from build123d import *

# Parameters (mm, degrees)
CROQUIS1_R                   = 275
SALIENTE_EXTRUIR1_DEPTH      = 70
CROQUIS2_R                   = 200
CORTAR_EXTRUIR1_DEPTH        = 40
CROQUIS5_R                   = 10
CORTAR_EXTRUIR2_DEPTH        = 10
REDONDEO1_R                  = 2
CORTAR_EXTRUIR_L_MINA2_DEPTH = 396.15819617
MATRIZC1_COUNT               = 24
CORTAR_EXTRUIR3_DEPTH        = 150
SALIENTE_EXTRUIR2_DEPTH      = 50
SALIENTE_EXTRUIR2_DEPTH_BACK = 50
CROQUIS12_R                  = 19.934957438
CROQUIS14_R                  = 285.546784005
CROQUIS14_R_2                = 202
SALIENTE_EXTRUIR3_DEPTH      = 100
REDONDEO2_R                  = 30
REDONDEO3_R                  = 30
SCALE1_SCALE                 = 0.5
SCALE2_SCALE                 = 0.1
SCALE3_SCALE                 = 0.2
SCALE4_SCALE                 = 0.3
SCALE5_SCALE                 = 20
SCALE6_SCALE                 = 1.5
SKETCH1_R                    = 1
CUT_EXTRUDE1_DEPTH           = 5


with BuildPart() as part:
    # Croquis1 → Saliente-Extruir1 (new body)
    with BuildSketch(Plane.XY):
        Circle(CROQUIS1_R)
    extrude(amount=SALIENTE_EXTRUIR1_DEPTH)

    # Croquis2 → Cortar-Extruir1 (cut)
    with BuildSketch(Plane.XY.offset(70)):
        Circle(CROQUIS2_R)
    extrude(amount=-CORTAR_EXTRUIR1_DEPTH, mode=Mode.SUBTRACT)

    # Croquis5 → Cortar-Extruir2 (cut)
    with BuildSketch(Plane.XY.offset(30)):
        Circle(CROQUIS5_R)
    extrude(amount=-CORTAR_EXTRUIR2_DEPTH, mode=Mode.SUBTRACT)

    # Redondeo1
    redondeo1_edges = [part.edges().sort_by_distance(p)[0] for p in [
        (-200, 0, 70),
    ]]
    fillet(redondeo1_edges, radius=REDONDEO1_R)

    # Croquis6 → Cortar-Extruir-Lámina2 (cut, through all)
    with BuildSketch(Plane.XY.offset(70)):
        Polygon((-99.341458201, 256.429863086), (-89.226691548, 230.320640663), (-89.319938771, 230.284516496), (-99.434705424, 256.39373892), align=None)
    cortar_extruir_l_mina2 = extrude(amount=-CORTAR_EXTRUIR_L_MINA2_DEPTH, mode=Mode.SUBTRACT)

    # MatrizC1: Cortar-Extruir-Lámina2 ×24 about axis
    matrizc1_axis = Axis((0, 0, 0), (0, 0, 1))
    for i in range(1, MATRIZC1_COUNT):
        add(cortar_extruir_l_mina2.rotate(matrizc1_axis, i * 360 / MATRIZC1_COUNT), mode=Mode.SUBTRACT)

    # Croquis11 → Cortar-Extruir3 (cut)
    with BuildSketch(Plane.XY.offset(30)):
        with BuildLine():
            Line((-13.902980207, 16.854693372), (-118.639144382, 161.011656163))
            ThreePointArc((-118.639144382, 161.011656163), (-161.803398875, 117.557050458), (-189.792696605, 63.077193306))
            Line((-189.792696605, 63.077193306), (-20.326023118, 8.014133235))
            ThreePointArc((-20.326023118, 8.014133235), (-17.676115044, 12.842449309), (-13.902980207, 16.854693372))
        make_face()
        with BuildLine():
            Line((-1.340807064, 21.807700102), (-1.340807064, 199.995505541))
            ThreePointArc((-1.340807064, 199.995505541), (-61.803398875, 190.211303259), (-116.469672981, 162.587869399))
            Line((-116.469672981, 162.587869399), (-11.733508805, 18.430906609))
            ThreePointArc((-11.733508805, 18.430906609), (-6.751675158, 20.779519481), (-1.340807064, 21.807700102))
        make_face()
        with BuildLine():
            Line((11.733508805, 18.430906609), (116.469672981, 162.587869399))
            ThreePointArc((116.469672981, 162.587869399), (61.803398875, 190.211303259), (1.340807064, 199.995505541))
            Line((1.340807064, 199.995505541), (1.340807064, 21.807700102))
            ThreePointArc((1.340807064, 21.807700102), (6.751675158, 20.779519481), (11.733508805, 18.430906609))
        make_face()
        with BuildLine():
            Line((20.326023118, 8.014133235), (189.792696605, 63.077193306))
            ThreePointArc((189.792696605, 63.077193306), (161.803398875, 117.557050458), (118.639144382, 161.011656163))
            Line((118.639144382, 161.011656163), (13.902980207, 16.854693372))
            ThreePointArc((13.902980207, 16.854693372), (17.676115044, 12.842449309), (20.326023118, 8.014133235))
        make_face()
        with BuildLine():
            ThreePointArc((200, 0), (197.641433142, 30.624563763), (190.621360943, 60.526826715))
            Line((190.621360943, 60.526826715), (21.154687456, 5.463766645))
            ThreePointArc((21.154687456, 5.463766645), (21.674636908, 2.75384499), (21.848879772, 0))
            ThreePointArc((21.848879772, 0), (21.674636908, -2.75384499), (21.154687456, -5.463766645))
            Line((21.154687456, -5.463766644), (190.621360943, -60.526826715))
            ThreePointArc((190.621360943, -60.526826715), (197.641433142, -30.624563763), (200, 0))
        make_face()
        with BuildLine():
            ThreePointArc((118.639144382, -161.011656163), (161.803398875, -117.557050458), (189.792696605, -63.077193306))
            Line((189.792696605, -63.077193306), (20.326023118, -8.014133235))
            ThreePointArc((20.326023118, -8.014133235), (17.676115044, -12.842449309), (13.902980207, -16.854693372))
            Line((13.902980207, -16.854693372), (118.639144382, -161.011656163))
        make_face()
        with BuildLine():
            Line((-21.154687456, 5.463766645), (-190.621360943, 60.526826715))
            ThreePointArc((-190.621360943, 60.526826715), (-200, 0), (-190.621360943, -60.526826715))
            Line((-190.621360943, -60.526826715), (-21.154687456, -5.463766644))
            ThreePointArc((-21.154687456, -5.463766644), (-21.848879772, 0), (-21.154687456, 5.463766645))
        make_face()
        with BuildLine():
            ThreePointArc((-189.792696605, -63.077193306), (-161.803398875, -117.557050458), (-118.639144382, -161.011656163))
            Line((-118.639144382, -161.011656163), (-13.902980207, -16.854693372))
            ThreePointArc((-13.902980207, -16.854693372), (-17.676115044, -12.842449309), (-20.326023118, -8.014133235))
            Line((-20.326023118, -8.014133235), (-189.792696605, -63.077193306))
        make_face()
        with BuildLine():
            ThreePointArc((-116.469672981, -162.587869399), (-61.803398875, -190.211303259), (-1.340807064, -199.995505541))
            Line((-1.340807064, -199.995505541), (-1.340807064, -21.807700102))
            ThreePointArc((-1.340807064, -21.807700102), (-6.751675158, -20.779519481), (-11.733508805, -18.430906609))
            Line((-11.733508805, -18.430906609), (-116.469672981, -162.587869399))
        make_face()
        with BuildLine():
            ThreePointArc((1.340807064, -199.995505541), (61.803398875, -190.211303259), (116.469672981, -162.587869399))
            Line((116.469672981, -162.587869399), (11.733508805, -18.430906609))
            ThreePointArc((11.733508805, -18.430906609), (6.751675158, -20.779519481), (1.340807064, -21.807700102))
            Line((1.340807064, -21.807700102), (1.340807064, -199.995505541))
        make_face()
    extrude(amount=-CORTAR_EXTRUIR3_DEPTH, mode=Mode.SUBTRACT)

    # Croquis12 → Saliente-Extruir2 (add, two sides: drawn at the far end of the back side and taken through both)
    with BuildSketch(Plane.XY.offset(20).offset(-SALIENTE_EXTRUIR2_DEPTH_BACK)):
        Circle(CROQUIS12_R)
    extrude(amount=SALIENTE_EXTRUIR2_DEPTH + SALIENTE_EXTRUIR2_DEPTH_BACK)

    # Croquis14 → Saliente-Extruir3 (add)
    with BuildSketch(Plane.XY.offset(70)):
        Circle(CROQUIS14_R)
        Circle(CROQUIS14_R_2, mode=Mode.SUBTRACT)
    extrude(amount=-SALIENTE_EXTRUIR3_DEPTH)

    # Redondeo2
    redondeo2_edges = [part.edges().sort_by_distance(p)[0] for p in [
        (-285.546784005, 0, 70),
    ]]
    fillet(redondeo2_edges, radius=REDONDEO2_R)

    # Redondeo3
    redondeo3_edges = [part.edges().sort_by_distance(p)[0] for p in [
        (-285.546784005, 0, -30),
    ]]
    fillet(redondeo3_edges, radius=REDONDEO3_R)


with BuildPart() as part_1:
    # Scale1: scaled about (0, 0, 20.146701312)
    add(part.part.scale(SCALE1_SCALE).moved(Location((0, 0, 10.073350656))))


with BuildPart() as part_2:
    # Scale2: scaled about (0, 0, 20.146701312)
    add(part_1.part.scale(SCALE2_SCALE).moved(Location((0, 0, 18.132031181))))


with BuildPart() as part_3:
    # Scale3: scaled about (0, 0, 20.146701312)
    add(part_2.part.scale(SCALE3_SCALE).moved(Location((0, 0, 16.11736105))))


with BuildPart() as part_4:
    # Scale4: scaled about (0, 0, 20.146701312)
    add(part_3.part.scale(SCALE4_SCALE).moved(Location((0, 0, 14.102690918))))


with BuildPart() as part_5:
    # Scale5: scaled about (0, 0, 20.146701312)
    add(part_4.part.scale(SCALE5_SCALE).moved(Location((0, 0, -382.787324928))))


with BuildPart() as part_6:
    # Scale6: scaled about (0, 0, 20.146701312)
    add(part_5.part.scale(SCALE6_SCALE).moved(Location((0, 0, -10.073350656))))

    # Sketch1 → Cut-Extrude1 (cut)
    with BuildSketch(Plane.XY.offset(24.633498194)):
        Circle(SKETCH1_R)
    extrude(amount=-CUT_EXTRUDE1_DEPTH, mode=Mode.SUBTRACT)


solid = part_6.part
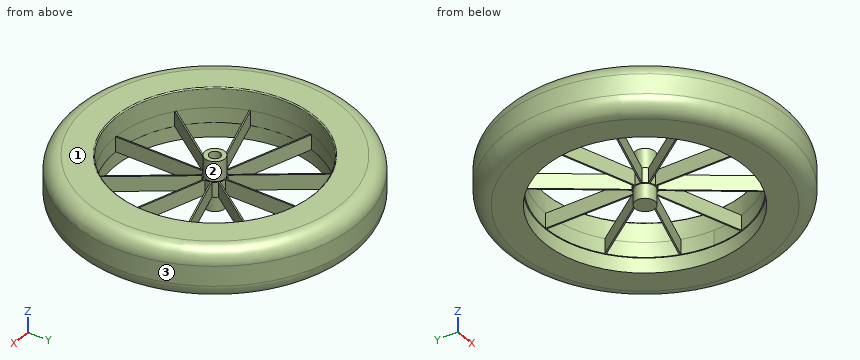
Can you work these out from the model? Positions are in its coordinate system, mm. Face numbers are marked on the shaded views. Coordinates: 2 decimals unless noted, no trailing zeros. Loops run counter-clockwise (first coordinate to the right, second up) from the corner with the lowest first, then second, coordinate; pieces in that order, holes last. Notation, with made-up numbers: (70, -9) - (86, -9) arc R21 cw to (86, 25) - close; hole circle Ø11 at (39, 77.5). An arc over 180 degrees is marked (long way). Put each result on its own line as item: value. Start each with the question number.
Item 1: If we mould it in two halves opening along Y, with no side actions, what happens to the marked faces 1, 2 and 3? For each: +Y half, -Y half, draft (parallel to the pull), parting line (faces both ways), or undercut.
Item 2: Suppose I cut it at D-D (z = 23). Please give me the cut outline in (x, y), and give its area (3 significant figures).
Item 3: For pin 1 (1.4 mm diameter, centred on y = -13, z = 19, fed in from -X); pin 2 (1.5 mm diameter, centred on y = 16.5, z = 17, fed in from +X); pin 3 (2 mm diameter, centred on x = -6, z = 18.5, fed in from -Y), each with a flat end and sliding along its axis, tell me the tip position at first contact or that it passes through.
Item 4: If I drill on line 1 along Y through (x, z) = (0, 16.7); line 2 along X through (y, z) = (-9, 19.75); line 3 along Y through (x, z) = (0, 21.85), over which ranges is the centre line in solid material (lowest first)?
Item 5: Suppose I cut it at A-A (z = 17.5). Please give me the cut outline in (x, y), and give its area (3 significant figures).
Item 6: Suppose I cut it at B-B (y = 4). State how many separate pieces and enclosed holes the cut face has, and give its area (3 significant figures).
Here are the results:
1. face 1: draft
1. face 2: undercut
1. face 3: parting line
2. outline: circle Ø50.96 at (0, 0); circle Ø3.59 at (0, 0); hole circle Ø36 at (0, 0); hole circle Ø2 at (0, 0)
2. area: 1,030 mm²
3. pin 1: x = -22.56
3. pin 2: x = 20.01
3. pin 3: y = -25.21
4. line 1: -25.15 to -18.18, -1.79 to 1.79, 18.18 to 25.15
4. line 2: -24.07 to -15.59, -6.69 to -6.39, -0.12 to 0.12, 6.39 to 6.69, 15.59 to 24.07
4. line 3: -25.7 to -18, -1.79 to -1, 1 to 1.79, 18 to 25.7
5. outline: circle Ø51.13 at (0, 0); circle Ø3.59 at (0, 0); hole circle Ø36.36 at (0, 0)
5. area: 1,030 mm²
6. separate pieces: 7
6. enclosed holes: 0
6. area: 140 mm²
